```python
from build123d import *

# Parameters (mm, degrees)
F0_W     = 3
F0_H     = 30
F1_DEPTH = 52.5
F3_DEPTH = 25
F5_DEPTH = 25
F6_R     = 2


with BuildPart() as f1:
    # F0 (on Top) → F1 (new body)
    with BuildSketch(Plane.XY):
        with Locations((-1.5, 15)):
            Rectangle(F0_W, F0_H)
        with Locations((-7.6, 15)):
            Rectangle(F0_W, F0_H)
        Polygon((40, 0), (0, 0), (-3, 0), (-6.1, 0), (-9.1, 0), (-9.1, -2.9952730983), (40, -3), align=None)
    extrude(amount=F1_DEPTH)

    # F2 (on face) → F3 (cut)
    with BuildSketch(Plane(origin=(-9.1, 0, 0), x_dir=(0, -1, 0), z_dir=(-1, 0, 0))):
        with BuildLine():
            Line((-13.5023634508, 37.5), (-13.5023634508, 39.25))
            ThreePointArc((-13.5023634508, 39.25), (-15.2523634508, 37.5), (-13.5023634508, 35.75))
            Line((-13.5023634508, 35.75), (-13.5023634508, 37.5))
        make_face()
        with BuildLine():
            ThreePointArc((-11.7523634508, 37.5), (-12.2649265837, 38.7374368671), (-13.5023634508, 39.25))
            Line((-13.5023634508, 39.25), (-13.5023634508, 37.5))
            Line((-13.5023634508, 37.5), (-13.5023634508, 35.75))
            ThreePointArc((-13.5023634508, 35.75), (-12.2649265837, 36.2625631329), (-11.7523634508, 37.5))
        make_face()
        with BuildLine():
            Line((-13.5023634508, 15), (-13.5023634508, 13.25))
            ThreePointArc((-13.5023634508, 13.25), (-12.2649265837, 13.7625631329), (-11.7523634508, 15))
            ThreePointArc((-11.7523634508, 15), (-12.2649265837, 16.2374368671), (-13.5023634508, 16.75))
            Line((-13.5023634508, 16.75), (-13.5023634508, 15))
        make_face()
        with BuildLine():
            ThreePointArc((-13.5023634508, 16.75), (-15.2523634508, 15), (-13.5023634508, 13.25))
            Line((-13.5023634508, 13.25), (-13.5023634508, 15))
            Line((-13.5023634508, 15), (-13.5023634508, 16.75))
        make_face()
    extrude(amount=-F3_DEPTH, mode=Mode.SUBTRACT)

    # F4 (on face) → F5 (cut)
    with BuildSketch(Plane(origin=(0, 0, 0), x_dir=(-1, 0, 0), z_dir=(0, 1, 0))):
        with BuildLine():
            ThreePointArc((-30, 37.75), (-28.7625631329, 38.2625631329), (-28.25, 39.5))
            Line((-28.25, 39.5), (-30, 39.5))
            Line((-30, 39.5), (-30, 37.75))
        make_face()
        with BuildLine():
            ThreePointArc((-28.25, 39.5), (-28.7625631329, 40.7374368671), (-30, 41.25))
            Line((-30, 41.25), (-30, 39.5))
            Line((-30, 39.5), (-28.25, 39.5))
        make_face()
        with BuildLine():
            Line((-30, 39.5), (-30, 41.25))
            ThreePointArc((-30, 41.25), (-31.2374368671, 40.7374368671), (-31.75, 39.5))
            Line((-31.75, 39.5), (-30, 39.5))
        make_face()
        with BuildLine():
            Line((-30, 37.75), (-30, 39.5))
            Line((-30, 39.5), (-31.75, 39.5))
            ThreePointArc((-31.75, 39.5), (-31.2374368671, 38.2625631329), (-30, 37.75))
        make_face()
        with BuildLine():
            Line((-10, 37.75), (-10, 39.5))
            Line((-10, 39.5), (-11.75, 39.5))
            ThreePointArc((-11.75, 39.5), (-11.2374368671, 38.2625631329), (-10, 37.75))
        make_face()
        with BuildLine():
            ThreePointArc((-10, 37.75), (-8.7625631329, 38.2625631329), (-8.25, 39.5))
            Line((-8.25, 39.5), (-10, 39.5))
            Line((-10, 39.5), (-10, 37.75))
        make_face()
        with BuildLine():
            ThreePointArc((-8.25, 39.5), (-8.7625631329, 40.7374368671), (-10, 41.25))
            Line((-10, 41.25), (-10, 39.5))
            Line((-10, 39.5), (-8.25, 39.5))
        make_face()
        with BuildLine():
            Line((-10, 39.5), (-10, 41.25))
            ThreePointArc((-10, 41.25), (-11.2374368671, 40.7374368671), (-11.75, 39.5))
            Line((-11.75, 39.5), (-10, 39.5))
        make_face()
        with BuildLine():
            Line((-10, 13), (-10, 14.75))
            ThreePointArc((-10, 14.75), (-11.2374368671, 14.2374368671), (-11.75, 13))
            Line((-11.75, 13), (-10, 13))
        make_face()
        with BuildLine():
            ThreePointArc((-8.25, 13), (-8.7625631329, 14.2374368671), (-10, 14.75))
            Line((-10, 14.75), (-10, 13))
            Line((-10, 13), (-8.25, 13))
        make_face()
        with BuildLine():
            ThreePointArc((-10, 11.25), (-8.7625631329, 11.7625631329), (-8.25, 13))
            Line((-8.25, 13), (-10, 13))
            Line((-10, 13), (-10, 11.25))
        make_face()
        with BuildLine():
            Line((-10, 11.25), (-10, 13))
            Line((-10, 13), (-11.75, 13))
            ThreePointArc((-11.75, 13), (-11.2374368671, 11.7625631329), (-10, 11.25))
        make_face()
        with BuildLine():
            ThreePointArc((-30, 11.25), (-28.7625631329, 11.7625631329), (-28.25, 13))
            Line((-28.25, 13), (-30, 13))
            Line((-30, 13), (-30, 11.25))
        make_face()
        with BuildLine():
            Line((-30, 13), (-31.75, 13))
            ThreePointArc((-31.75, 13), (-31.2374368671, 11.7625631329), (-30, 11.25))
            Line((-30, 11.25), (-30, 13))
        make_face()
        with BuildLine():
            Line((-30, 13), (-30, 14.75))
            ThreePointArc((-30, 14.75), (-31.2374368671, 14.2374368671), (-31.75, 13))
            Line((-31.75, 13), (-30, 13))
        make_face()
        with BuildLine():
            ThreePointArc((-28.25, 13), (-28.7625631329, 14.2374368671), (-30, 14.75))
            Line((-30, 14.75), (-30, 13))
            Line((-30, 13), (-28.25, 13))
        make_face()
        with BuildLine():
            Line((-20, 24.5), (-20, 26.25))
            Line((-20, 26.25), (-21.75, 26.25))
            ThreePointArc((-21.75, 26.25), (-21.2374368671, 25.0125631329), (-20, 24.5))
        make_face()
        with BuildLine():
            ThreePointArc((-20, 24.5), (-18.7625631329, 25.0125631329), (-18.25, 26.25))
            Line((-18.25, 26.25), (-20, 26.25))
            Line((-20, 26.25), (-20, 24.5))
        make_face()
        with BuildLine():
            ThreePointArc((-18.25, 26.25), (-18.7625631329, 27.4874368671), (-20, 28))
            Line((-20, 28), (-20, 26.25))
            Line((-20, 26.25), (-18.25, 26.25))
        make_face()
        with BuildLine():
            Line((-20, 26.25), (-20, 28))
            ThreePointArc((-20, 28), (-21.2374368671, 27.4874368671), (-21.75, 26.25))
            Line((-21.75, 26.25), (-20, 26.25))
        make_face()
    extrude(amount=-F5_DEPTH, mode=Mode.SUBTRACT)

    # F6
    f6_edges = [f1.edges().sort_by_distance(p)[0] for p in [
        (40, -1.5, 52.5),
        (-9.1, 30, 26.25),
        (-9.1, 13.502363, 52.5),
        (-7.6, 30, 52.5),
    ]]
    fillet(f6_edges, radius=F6_R)


solid = f1.part
```
Read the model definition and answer for the solid it produces. Units are mm, in the model's axes. A direction names the side the tool comes from. Coordinates: 2 decimals unless noted, no trailing zeros. Order: outer loops, then holes, each group sorted by start corner. A loop starts at its lowest first (then second) coordinate and runs counter-clockwise, first axis right, second up. Notation, with made-up numbers: (75.5, 40.5) - (82.5, 40.5) arc R32 cw to (82.5, 79.5) - close; hole circle Ø11 at (-37, 6.25). An arc over 180 degrees is marked (long way). Answer as a JSON object with one key per item and string values. Group by question number.
Item 1: Section B-B (z = 9) is taken. Give the vertices of the cut face in (x, y), plus the area to 3 significant figures.
Item 2: Section A-A (y = 6.5) is taken. Give the vertices of the cut face in (x, z).
Item 3: Consider probe 1 along X at (y, z) = (23.5, 34); probe 2 along Y at (x, z) = (29, 3); probe 3 along X at (y, z) = (29.5, 42.5). Determine where each line is inside the solid, lowest interval first. Write a range as from..to.
Item 4: A tool of negligible diameter and unlimited length cuts with its end or side. For faces 1 (the face through (-6.59, 29.4, 51.93)), 2 (the face through (39.4, -1.48, 51.93)), 3 (the face through (-5, 0, 26)), from which of +Z, -Z, +X, -X, +Y, -Y can it reach the whole face along a straight path? Write none if from no direction.
Item 5: Section C-C (x = 5) is taken. Give the vertices of the cut face in (y, z).
Item 6: Flat-ended cylindrical pins translate along their axes: P1, Ø5, axis at x = 9.5, z = 23.5, coming from the +Y side; P2, Ø3, axis at x = 6.5, z = 46, coming from the -Y side; P3, Ø2, axis at x = -2, y = 25.5, coming from the -Z side. Find the tip coordinate at first contact, or state that the pin passes through.
Item 7: The mould has two halves that part along X. Classify faces 4 (the face through (-6.1, 15, 26)), 5 (the face through (0, 15, 26)), 6 (the face through (-3, 15, 26)), 7 (the face through (16, 0, 26)): +X half, -X half, draft (parallel to the pull), parting line (faces both ways), or undercut.
Results are:
{
 "1": {"outline": "(-9.1, -3) - (40, -3) - (40, 0) - (0, 0) - (0, 30) - (-3, 30) - (-3, 0) - (-6.1, 0) - (-6.1, 30) - (-7.1, 30) arc R2 ccw to (-9.1, 28) - close", "area": "326 mm^2"},
 "2": {"outline": "(-9.1, 0) - (-6.1, 0) - (-6.1, 52.5) - (-7.1, 52.5) arc R2 ccw to (-9.1, 50.5) - close; (-3, 0) - (0, 0) - (0, 52.5) - (-3, 52.5) - close"},
 "3": {"probe 1": "x = -9.1..-6.1, -3..0", "probe 2": "y = -3..0", "probe 3": "x = -8.42..-6.1, -3..0"},
 "4": {"face 1": "+Z, -X, +Y", "face 2": "+Z, +X, +Y, -Y", "face 3": "+Z, -Z, +Y"},
 "5": {"outline": "(-3, 0) - (0, 0) - (0, 52.5) - (-3, 52.5) - close"},
 "6": {"P1": "stops at y = 0", "P2": "stops at y = -3", "P3": "stops at z = 0"},
 "7": {"face 4": "undercut", "face 5": "+X half", "face 6": "undercut", "face 7": "draft"}
}
